from build123d import *

# Parameters (mm, degrees)
SKETCH_W                       = 55
SKETCH_H                       = 60
PAD_DEPTH                      = 11
SKETCH001_R                    = 7.6
POCKET_DEPTH                   = 60.001
SKETCH002_R                    = 1.75
POCKET001_DEPTH                = 11.001
POCKET002_DEPTH                = 9
SKETCH004_R                    = 2.25
POCKET003_DEPTH                = 11.001
SKETCH008_R                    = 4.1
POCKET005_DEPTH                = 20
SKETCH010_W                    = 20
SKETCH010_H                    = 25
POCKET006_DEPTH                = 5
CHAMFER_SIZE                   = 3
CHAMFER001_SIZE                = 3
PART_MIRRORING_PLACEMENT_ANGLE = 180


with BuildPart() as chamfer002:
    # Sketch → Pad (new body)
    with BuildSketch(Plane.XY):
        with Locations((17.5, 0)):
            Rectangle(SKETCH_W, SKETCH_H)
    extrude(amount=PAD_DEPTH)

    # Sketch001 → Pocket (cut, through all)
    with BuildSketch(Plane.XZ.offset(30)):
        with Locations((0, 11)):
            Circle(SKETCH001_R)
    extrude(amount=-POCKET_DEPTH, mode=Mode.SUBTRACT)

    # Sketch002 → Pocket001 (cut, through all)
    with BuildSketch(Plane(origin=(0, 0, 0), x_dir=(1, 0, 0), z_dir=(0, 0, -1))):
        with Locations((-6, 27)):
            Circle(SKETCH002_R)
        with Locations((36, 27)):
            Circle(SKETCH002_R)
        with Locations((-6, -27)):
            Circle(SKETCH002_R)
        with Locations((36, -27)):
            Circle(SKETCH002_R)
        with Locations((6, 27)):
            Circle(SKETCH002_R)
        with Locations((6, -27)):
            Circle(SKETCH002_R)
        with Locations((6, 0)):
            Circle(SKETCH002_R)
        with Locations((-6, 0)):
            Circle(SKETCH002_R)
        with Locations((36, -13)):
            Circle(SKETCH002_R)
        with Locations((36, 13)):
            Circle(SKETCH002_R)
    extrude(amount=-POCKET001_DEPTH, mode=Mode.SUBTRACT)

    # Sketch003 → Pocket002 (cut)
    with BuildSketch(Plane.XY.offset(11)):
        with BuildLine():
            Line((10, 35), (10, -35))
            Line((10, -35), (28, -35))
            Line((28, -35), (28, -14.916198))
            ThreePointArc((28, -14.916198), (30.841983, -12.965458), (32.599342, -10))
            Line((32.599342, -10), (52.599342, -10))
            Line((52.599342, -10), (52.599342, 10))
            Line((52.599342, 10), (32.599342, 10))
            ThreePointArc((32.599342, 10), (30.841983, 12.965458), (28, 14.916198))
            Line((28, 14.916198), (28, 35))
            Line((28, 35), (10, 35))
        make_face()
    extrude(amount=-POCKET002_DEPTH, mode=Mode.SUBTRACT)

    # Sketch004 → Pocket003 (cut, through all)
    with BuildSketch(Plane(origin=(0, 0, 0), x_dir=(1, 0, 0), z_dir=(0, 0, -1))):
        with Locations((25, 7.5)):
            Circle(SKETCH004_R)
        with Locations((25, -7.5)):
            Circle(SKETCH004_R)
    extrude(amount=-POCKET003_DEPTH, mode=Mode.SUBTRACT)

    # Sketch008 → Pocket005 (cut)
    with BuildSketch(Plane.YZ.offset(45)):
        with Locations((-20, 11)):
            Circle(SKETCH008_R)
        with Locations((20, 11)):
            Circle(SKETCH008_R)
    extrude(amount=-POCKET005_DEPTH, mode=Mode.SUBTRACT)

    # Sketch010 → Pocket006 (cut)
    with BuildSketch(Plane.YZ.offset(45)):
        with Locations((0, 3.5)):
            Rectangle(SKETCH010_W, SKETCH010_H)
    extrude(amount=-POCKET006_DEPTH, mode=Mode.SUBTRACT)

    # Chamfer
    chamfer_edges = [chamfer002.edges().sort_by_distance(p)[0] for p in [
        (45, -10, 6.5),
    ]]
    chamfer(chamfer_edges, length=CHAMFER_SIZE)

    # Chamfer001
    chamfer001_edges = [chamfer002.edges().sort_by_distance(p)[0] for p in [
        (45, 10, 6.5),
    ]]
    chamfer(chamfer001_edges, length=CHAMFER001_SIZE)


with BuildPart() as xy_block_top:
    # Part__Mirroring: instance of Chamfer002
    add(chamfer002.part.mirror(Plane(origin=(0, 0, 0), x_dir=(0, 1, 0), z_dir=(0, 0, 1))))


with BuildPart() as xy_block_top_1:
    # Part__Mirroring placement: moved
    add(xy_block_top.part.rotate(Axis((0, 0, 0), (1, 0, 0)), PART_MIRRORING_PLACEMENT_ANGLE))


solid = xy_block_top_1.part
For this review, take the finished solid that the model builds, in its own axes (mm). A direction names the side the tool comes from. Round coordinates to 2 decimals unless told otherwise and drop trailing zeros. Loops run counter-clockwise (first coordinate to the right, second up) from the corner with the lowest first, then second, coordinate; pieces in that order, holes last. Notation, with made-up numbers: (-13.75, 86.25) - (4.25, 86.25) arc R14 cw to (4.25, 98.25) - close; hole circle Ø9 at (-15.5, 52.5). An arc over 180 degrees is marked (long way). Use one line per item in the form item = value.
Item 1: Consider section C-C on z = 10. State how many separate pieces and enclosed holes the cut face has, then the cut area to 3 significant figures.
Answers:
separate_pieces = 6
enclosed_holes = 4
area = 627 mm^2
Item 2: Mouldability with a two-part tool opening along X and no side actions: class faces 1 (the cylindrical face through (30.81, 13, 6.56)), 2 (the flat face through (38, 27, 11)), 3 (the flat face through (40, 0, 1)) as +X half, -X half, draft (parallel to the pull), parting line (faces both ways), or undercut.
Answers:
face_1 = undercut
face_2 = draft
face_3 = +X half
Item 3: Consider section A-A on y = -7.5. Write out the cut boundary in (x, z), then the cut area to 3 significant figures.
Answers:
outline = (-10, 0) - (22.75, 0) - (22.75, 2) - (10, 2) - (10, 11) - (7.6, 11) arc R7.6 cw to (-7.6, 11) - (-10, 11) - close; (27.25, 0) - (40, 0) - (40, 2) - (27.25, 2) - close
area = 180 mm^2
Item 4: Consider section D-D on x = -6. Write out the cut boundary in (y, z), then the cut area to 3 significant figures.
Answers:
outline = (-30, 0) - (-28.75, 0) - (-28.75, 6.34) - (-30, 6.34) - close; (-25.25, 0) - (-1.75, 0) - (-1.75, 6.34) - (-25.25, 6.34) - close; (1.75, 0) - (25.25, 0) - (25.25, 6.34) - (1.75, 6.34) - close; (28.75, 0) - (30, 0) - (30, 6.34) - (28.75, 6.34) - close
area = 314 mm^2
Item 5: For line 1 (Y direction, x = -6, z = 5.5); line 2 (X direction, y = -20.5, z = 5.5) (3 decimals); line 3 (X direction, y = 0, z = 7), list the stretches that pass through material, from the lowest coordinate up.
Answers:
line_1 = -30 to -28.75, -25.25 to -1.75, 1.75 to 25.25, 28.75 to 30
line_2 = -10 to -5.245, 5.245 to 10, 28 to 45
line_3 = -10 to -7.75, 7.75 to 10
Item 6: Tool access review of faces 4 (the flat face through (28, 23, 6)), 5 (the cylindrical face through (30.9, -12.9, 6.6)), 6 (the cylindrical face through (36.6, 20.1, 6.9)): name each direction out of +Z, -Z, +X, -X, +Y, -Y from which nothing blocks a thin tool from reaching the whole face with its end or side.
Answers:
face_4 = +Z, +Y, -Y
face_5 = +Z
face_6 = +Z, +X
Item 7: Clearance check with flat-ended pins moving along their axes: P1, Ø3.5, axis at x = 25, y = -7.5, coming from the +Z side; P2, Ø3, axis at x = 1, y = 23.5, coming from the +Z side. State where each tip first meets the part, or that it passes through.
Answers:
P1 = through
P2 = 3.82
Item 8: Consider section B-B on y = 0. Write out the cut boundary in (x, z), then the cut area to 3 significant figures.
Answers:
outline = (-10, 0) - (-7.75, 0) - (-7.75, 11) - (-10, 11) - close; (-4.25, 0) - (4.25, 0) - (4.25, 4.7) arc R7.6 cw to (-4.25, 4.7) - close; (7.75, 0) - (40, 0) - (40, 2) - (10, 2) - (10, 11) - (7.75, 11) - close
area = 142 mm^2
